```python
from build123d import *

# Parameters (mm, degrees)
SKETCH_2_R               = 20
EXTRUDE_3_DEPTH          = 4
CUT_EXTRUDE_6_DEPTH      = 5
CUT_EXTRUDE_6_DEPTH_BACK = 5
CUT_EXTRUDE_7_DEPTH      = 5
CUT_EXTRUDE_7_DEPTH_BACK = 5
EXTRUDE_4_DEPTH          = 4
EXTRUDE_5_DEPTH          = 4


with BuildPart() as part:
    # Эскиз2 → Бобышка-Вытянуть3 (new body, symmetric)
    with BuildSketch(Plane.XY):
        Circle(SKETCH_2_R)
    extrude(amount=EXTRUDE_3_DEPTH, both=True)

    # Эскиз2<10> → Вырез-Вытянуть6 (cut, two sides)
    with BuildSketch(Plane.XY) as cut_extrude_6_sk:
        with BuildLine():
            Line((-1.5612495, 1.55), (1.5612495, 1.55))
            ThreePointArc((1.5612495, 1.55), (0, -2.2), (-1.5612495, 1.55))
        make_face()
    extrude(amount=CUT_EXTRUDE_6_DEPTH, mode=Mode.SUBTRACT)
    extrude(cut_extrude_6_sk.sketch, amount=-CUT_EXTRUDE_6_DEPTH_BACK, mode=Mode.SUBTRACT)

    # Эскиз2<11> → Вырез-Вытянуть7 (cut, two sides)
    with BuildSketch(Plane.XY) as cut_extrude_7_sk:
        with BuildLine():
            ThreePointArc((13.856406461, 2), (9.899494937, 9.899494937), (2, 13.856406461))
            Line((2, 13.856406461), (2, 4.582575695))
            ThreePointArc((2, 4.582575695), (3.535533906, 3.535533906), (4.582575695, 2))
            Line((4.582575695, 2), (13.856406461, 2))
        make_face()
        with BuildLine():
            ThreePointArc((-2, 13.856406461), (-9.899494937, 9.899494937), (-13.856406461, 2))
            Line((-13.856406461, 2), (-4.582575695, 2))
            ThreePointArc((-4.582575695, 2), (-3.535533906, 3.535533906), (-2, 4.582575695))
            Line((-2, 4.582575695), (-2, 13.856406461))
        make_face()
        with BuildLine():
            Line((-4.582575695, -2), (-13.856406461, -2))
            ThreePointArc((-13.856406461, -2), (-9.899494937, -9.899494937), (-2, -13.856406461))
            Line((-2, -13.856406461), (-2, -4.582575695))
            ThreePointArc((-2, -4.582575695), (-3.535533906, -3.535533906), (-4.582575695, -2))
        make_face()
        with BuildLine():
            Line((2, -4.582575695), (2, -13.856406461))
            ThreePointArc((2, -13.856406461), (9.899494937, -9.899494937), (13.856406461, -2))
            Line((13.856406461, -2), (4.582575695, -2))
            ThreePointArc((4.582575695, -2), (3.535533906, -3.535533906), (2, -4.582575695))
        make_face()
    extrude(amount=CUT_EXTRUDE_7_DEPTH, mode=Mode.SUBTRACT)
    extrude(cut_extrude_7_sk.sketch, amount=-CUT_EXTRUDE_7_DEPTH_BACK, mode=Mode.SUBTRACT)

    # Эскиз2<12> → Бобышка-Вытянуть4 (add)
    with BuildSketch(Plane.XY):
        with BuildLine():
            ThreePointArc((20, 0), (19.960745185, -1.252458251), (19.843134833, -2.5))
            Line((19.843134833, -2.5), (39.843134833, -2.5))
            Line((39.843134833, -2.5), (39.843134833, 2.5))
            Line((39.843134833, 2.5), (19.843134833, 2.5))
            ThreePointArc((19.843134833, 2.5), (19.960745185, 1.252458251), (20, 0))
        make_face()
        with BuildLine():
            Line((26.405583871, 29.941117777), (12.263448247, 15.798982153))
            ThreePointArc((12.263448247, 15.798982153), (14.142135624, 14.142135624), (15.798982153, 12.263448247))
            Line((15.798982153, 12.263448247), (29.941117777, 26.405583871))
            Line((29.941117777, 26.405583871), (26.405583871, 29.941117777))
        make_face()
        with BuildLine():
            Line((-2.5, 39.843134833), (-2.5, 19.843134833))
            ThreePointArc((-2.5, 19.843134833), (0, 20), (2.5, 19.843134833))
            Line((2.5, 19.843134833), (2.5, 39.843134833))
            Line((2.5, 39.843134833), (-2.5, 39.843134833))
        make_face()
        with BuildLine():
            Line((-29.941117777, 26.405583871), (-15.798982153, 12.263448247))
            ThreePointArc((-15.798982153, 12.263448247), (-14.142135624, 14.142135624), (-12.263448247, 15.798982153))
            Line((-12.263448247, 15.798982153), (-26.405583871, 29.941117777))
            Line((-26.405583871, 29.941117777), (-29.941117777, 26.405583871))
        make_face()
        with BuildLine():
            Line((-39.843134833, -2.5), (-19.843134833, -2.5))
            ThreePointArc((-19.843134833, -2.5), (-20, 0), (-19.843134833, 2.5))
            Line((-19.843134833, 2.5), (-39.843134833, 2.5))
            Line((-39.843134833, 2.5), (-39.843134833, -2.5))
        make_face()
        with BuildLine():
            ThreePointArc((-12.263448247, -15.798982153), (-14.142135624, -14.142135624), (-15.798982153, -12.263448247))
            Line((-15.798982153, -12.263448247), (-29.941117777, -26.405583871))
            Line((-29.941117777, -26.405583871), (-26.405583871, -29.941117777))
            Line((-26.405583871, -29.941117777), (-12.263448247, -15.798982153))
        make_face()
        with BuildLine():
            ThreePointArc((2.5, -19.843134833), (0, -20), (-2.5, -19.843134833))
            Line((-2.5, -19.843134833), (-2.5, -39.843134833))
            Line((-2.5, -39.843134833), (2.5, -39.843134833))
            Line((2.5, -39.843134833), (2.5, -19.843134833))
        make_face()
        with BuildLine():
            ThreePointArc((15.798982153, -12.263448247), (14.142135624, -14.142135624), (12.263448247, -15.798982153))
            Line((12.263448247, -15.798982153), (26.405583871, -29.941117777))
            Line((26.405583871, -29.941117777), (29.941117777, -26.405583871))
            Line((29.941117777, -26.405583871), (15.798982153, -12.263448247))
        make_face()
    extrude(amount=EXTRUDE_4_DEPTH)

    # Эскиз2<13> → Бобышка-Вытянуть5 (add)
    with BuildSketch(Plane.XY):
        with BuildLine():
            Line((-17.557006425, 35.853548202), (-9.903337778, 17.375957552))
            ThreePointArc((-9.903337778, 17.375957552), (-7.653668647, 18.47759065), (-5.283940115, 19.289374714))
            Line((-5.283940115, 19.289374714), (-12.937608763, 37.766965364))
            Line((-12.937608763, 37.766965364), (-17.557006425, 35.853548202))
        make_face()
        with BuildLine():
            Line((-37.766965364, 12.937608763), (-19.289374714, 5.283940115))
            ThreePointArc((-19.289374714, 5.283940115), (-18.47759065, 7.653668647), (-17.375957552, 9.903337778))
            Line((-17.375957552, 9.903337778), (-35.853548202, 17.557006425))
            Line((-35.853548202, 17.557006425), (-37.766965364, 12.937608763))
        make_face()
        with BuildLine():
            ThreePointArc((-17.375957552, -9.903337778), (-18.47759065, -7.653668647), (-19.289374714, -5.283940115))
            Line((-19.289374714, -5.283940115), (-37.766965364, -12.937608763))
            Line((-37.766965364, -12.937608763), (-35.853548202, -17.557006425))
            Line((-35.853548202, -17.557006425), (-17.375957552, -9.903337778))
        make_face()
        with BuildLine():
            ThreePointArc((-5.283940115, -19.289374714), (-7.653668647, -18.47759065), (-9.903337778, -17.375957552))
            Line((-9.903337778, -17.375957552), (-17.557006425, -35.853548202))
            Line((-17.557006425, -35.853548202), (-12.937608763, -37.766965364))
            Line((-12.937608763, -37.766965364), (-5.283940115, -19.289374714))
        make_face()
        with BuildLine():
            ThreePointArc((9.903337778, -17.375957552), (7.653668647, -18.47759065), (5.283940115, -19.289374714))
            Line((5.283940115, -19.289374714), (12.937608763, -37.766965364))
            Line((12.937608763, -37.766965364), (17.557006425, -35.853548202))
            Line((17.557006425, -35.853548202), (9.903337778, -17.375957552))
        make_face()
        with BuildLine():
            ThreePointArc((19.289374714, -5.283940115), (18.47759065, -7.653668647), (17.375957552, -9.903337778))
            Line((17.375957552, -9.903337778), (35.853548202, -17.557006425))
            Line((35.853548202, -17.557006425), (37.766965364, -12.937608763))
            Line((37.766965364, -12.937608763), (19.289374714, -5.283940115))
        make_face()
        with BuildLine():
            Line((35.853548202, 17.557006425), (17.375957552, 9.903337778))
            ThreePointArc((17.375957552, 9.903337778), (18.47759065, 7.653668647), (19.289374714, 5.283940115))
            Line((19.289374714, 5.283940115), (37.766965364, 12.937608763))
            Line((37.766965364, 12.937608763), (35.853548202, 17.557006425))
        make_face()
        with BuildLine():
            Line((12.937608763, 37.766965364), (5.283940115, 19.289374714))
            ThreePointArc((5.283940115, 19.289374714), (7.653668647, 18.47759065), (9.903337778, 17.375957552))
            Line((9.903337778, 17.375957552), (17.557006425, 35.853548202))
            Line((17.557006425, 35.853548202), (12.937608763, 37.766965364))
        make_face()
    extrude(amount=-EXTRUDE_5_DEPTH)


solid = part.part
```
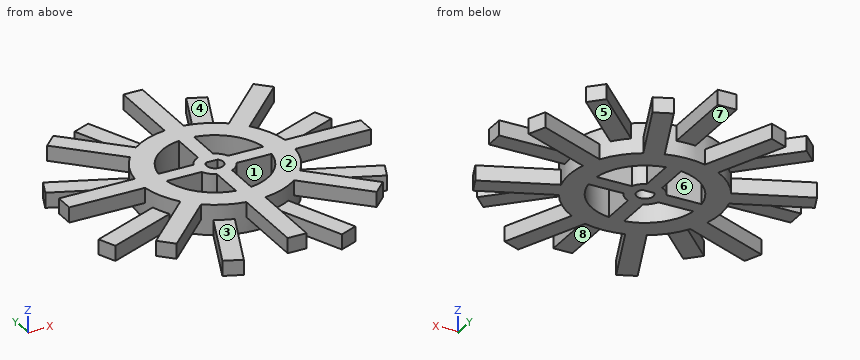
Can you work these out from the model? Positions are in its coordinate system, mm. Face numbers are marked on the shaded views. A direction names the side the tool comes from. Round coordinates to 2 decimals unless told otherwise and drop trailing zeros. Loops run counter-clockwise (first coordinate to the right, second up) from the corner with the lowest first, then second, coordinate; pieces in that order, holes last. Notation, with made-up numbers: (-3.5, -4) -> (35.5, -4) arc R15 ccw to (35.5, 11) -> close; hole circle Ø3 at (19, -9.75). An arc over 180 degrees is marked (long way). Answer in a Markdown table with one row per item.
Item 1: If I drill on probe 1 along Y at (x, z) = (0, 0.75); probe 2 along X at (y, z) = (0, 2.75); probe 3 along X at (y, z) = (28, 1), over which ranges is the centre line in solid material (lowest first)?
Answer block:
| item | result |
|---|---|
| probe 1 | -39.84 to -2.2, 1.55 to 39.84 |
| probe 2 | -39.84 to -2.2, 2.2 to 39.84 |
| probe 3 | -28.35 to -24.46, -2.5 to 2.5, 24.46 to 28.35 |
Item 2: We'd pull the mould along X, two halves only. Please class the marked faces 1, 2 and 3: released by +X, released by -X, zero draft, split by the parting line, or undercut.
Answer block:
| item | result |
|---|---|
| face 1 | undercut |
| face 2 | zero draft |
| face 3 | undercut |
Item 3: Suppose I cut it at D-D, the plane y = -23. List the corners of the cut face in (x, z) for me.
Answer block:
| item | result |
|---|---|
| outline | (-26.54, 0) -> (-19.46, 0) -> (-19.46, 4) -> (-26.54, 4) -> close; (-12.23, -4) -> (-6.82, -4) -> (-6.82, 0) -> (-12.23, 0) -> close; (-2.5, 0) -> (2.5, 0) -> (2.5, 4) -> (-2.5, 4) -> close; (6.82, -4) -> (12.23, -4) -> (12.23, 0) -> (6.82, 0) -> close; (19.46, 0) -> (26.54, 0) -> (26.54, 4) -> (19.46, 4) -> close |
Item 4: Suppose I cut it at C-C, the plane z = 1.5. Give the number of separate pieces and of enclosed holes in the cut face, plus the area to 3 significant figures.
Answer block:
| item | result |
|---|---|
| separate pieces | 1 |
| enclosed holes | 5 |
| area | 1,650 mm² |
Item 5: On a 3-axis mill with a long thin cutter (end or side, diameter ignored), from which of +Z, -Z, +X, -X, +Y, -Y can I reach the whole of each face in a straight line? I mean the marked faces 4, 5, 6, 7 and 8. Say none if no direction works.
Answer block:
| item | result |
|---|---|
| face 4 | +Z, +Y |
| face 5 | -Z |
| face 6 | +Z, -Z |
| face 7 | -Z, +Y |
| face 8 | -Z, -Y |
Item 6: Suppose I cut it at B-B, the plane x = 0. List the corners of the cut face in (y, z) for me.
Answer block:
| item | result |
|---|---|
| outline | (-39.84, 0) -> (-20, 0) -> (-20, -4) -> (-2.2, -4) -> (-2.2, 4) -> (-39.84, 4) -> close; (1.55, -4) -> (20, -4) -> (20, 0) -> (39.84, 0) -> (39.84, 4) -> (1.55, 4) -> close |
Item 7: Will these pins go through, and if not, where does the flat tip stop? P1, Ø2, axis at x = -27, z = 2.5, coming from the -Y side; P2, Ø2, axis at y = 32, z = 2, coming from the +X side; P3, Ø1.5, axis at x = -34, y = -1, coming from the -Z side; P4, Ø2, axis at x = -12.5, y = 19, coming from the -Z side.
Answer block:
| item | result |
|---|---|
| P1 | y = -29.94 |
| P2 | x = 2.5 |
| P3 | z = 0 |
| P4 | through |
Item 8: Suppose I cut it at A-A, the plane y = 0. List the corners of the cut face in (x, z) for me.
Answer block:
| item | result |
|---|---|
| outline | (-39.84, 0) -> (-20, 0) -> (-20, -4) -> (-2.2, -4) -> (-2.2, 4) -> (-39.84, 4) -> close; (2.2, -4) -> (20, -4) -> (20, 0) -> (39.84, 0) -> (39.84, 4) -> (2.2, 4) -> close |
